Design review of the part built by this model. Coordinates are the model's own, in mm. A direction names the side the tool comes from. Give positions to 0.01 mm unless a question says otherwise; leave off trailing zeros. Write each loop counter-clockwise with the first axis right and the second up, starting at its lowest first coordinate (ties: lowest second). Pieces come first, ordered by that corner, then holes. Notation, with made-up numbers: (13.25, 69.5) -> (31.25, 69.5) arc R17 cw to (31.25, 90.5) -> close; hole circle Ø8 at (65.5, 25). An arc over 180 degrees is marked (long way). Answer as a JSON object with one key per item and string values.
```python
from build123d import *


with BuildPart() as part:
    # Sweep2: sweep along a path in BasketRing
    with BuildLine(Plane.XY) as sweep2_path:
        Line((44, 0), (273.5, 0))
        ThreePointArc((273.5, 0), (304.612698372, 12.887301628), (317.5, 44))
        Line((317.5, 44), (317.5, 203.5))
        ThreePointArc((317.5, 203.5), (304.612698372, 234.612698372), (273.5, 247.5))
        Line((273.5, 247.5), (44, 247.5))
        ThreePointArc((44, 247.5), (12.887301628, 234.612698372), (0, 203.5))
        Line((0, 203.5), (0, 44))
        ThreePointArc((0, 44), (12.887301628, 12.887301628), (44, 0))
    # ShapeOf Edge → Sweep2 (sweep)
    with BuildSketch(Plane(origin=(44, 0, 0), x_dir=(0, 0, -1), z_dir=(1, 0, 0))):
        Polygon((0, 0), (2.4, 0), (2.4, -2.4), (70.4, -2.4), (70.4, 0), (5.854935695, 0), (2.748344754, 3), (0, 3), align=None)
    sweep(path=sweep2_path.line)


solid = part.part
```
(1) The part is to be moulded in two halves that separate along X. For faces 1 (the conical face through (15.227, 232.913, -2.899)), 2 (the cylindrical face through (304.27, 12.55, -37.68)), 3 (the flat face through (-2.4, 123, -36)), 4 (the cylindrical face through (304.95, 234.27, -1.22)), say which applies: +X half, -X half, draft (parallel to the pull), parting line (faces both ways), or undercut.
Here are the results:
{"face 1": "undercut", "face 2": "undercut", "face 3": "-X half", "face 4": "+X half"}
(2) We need section A-A, the plane y = 58.5. State the section outline as (x, z) points.
Here are the results:
{"outline": "(-2.4, -70.4) -> (0, -70.4) -> (0, -5.85) -> (3, -2.75) -> (3, 0) -> (0, 0) -> (0, -2.4) -> (-2.4, -2.4) -> close; (314.5, -2.75) -> (317.5, -5.85) -> (317.5, -70.4) -> (319.9, -70.4) -> (319.9, -2.4) -> (317.5, -2.4) -> (317.5, 0) -> (314.5, 0) -> close"}
(3) For faces 5 (the cylindrical face through (12.55, 13.23, -1.22)), 6 (the cylindrical face through (14.69, 15.33, -1.35)), 7 (the flat face through (160, 0, -39)), list the 3-axis set-ups (+Z, -Z, +X, -X, +Y, -Y) from which the entire face can be reached by the end or side of a thin tool; tool diameter is ignored.
Here are the results:
{"face 5": "+Z, -X, -Y", "face 6": "+Z, -Z", "face 7": "-Z"}
(4) Clearance check with flat-ended pins moving along their axes: pin 1 (0.7 mm diameter, centred on x = 125, z = -0.5, fed in from +Y); pin 2 (1.5 mm diameter, centred on y = 207.5, z = -61, fed in from -X); pin 3 (3 mm diameter, centred on y = 207, z = -29, fed in from -X). State where each tip first meets the part, or that it passes through.
Here are the results:
{"pin 1": "stops at y = 247.5", "pin 2": "stops at x = -2.29", "pin 3": "stops at x = -2.36"}
(5) We need section C-C, the plane z = -11. State the section outline as (x, y) points.
Here are the results:
{"outline": "(-2.4, 44) arc R46.4 ccw to (44, -2.4) -> (273.5, -2.4) arc R46.4 ccw to (319.9, 44) -> (319.9, 203.5) arc R46.4 ccw to (273.5, 249.9) -> (44, 249.9) arc R46.4 ccw to (-2.4, 203.5) -> close; hole (0, 44) arc R44 ccw to (44, 0) -> (273.5, 0) arc R44 ccw to (317.5, 44) -> (317.5, 203.5) arc R44 ccw to (273.5, 247.5) -> (44, 247.5) arc R44 ccw to (0, 203.5) -> close"}
(6) We need section B-B, the plane x = 169. State the section outline as (y, z) points.
Here are the results:
{"outline": "(-2.4, -70.4) -> (0, -70.4) -> (0, -5.85) -> (3, -2.75) -> (3, 0) -> (0, 0) -> (0, -2.4) -> (-2.4, -2.4) -> close; (244.5, -2.75) -> (247.5, -5.85) -> (247.5, -70.4) -> (249.9, -70.4) -> (249.9, -2.4) -> (247.5, -2.4) -> (247.5, 0) -> (244.5, 0) -> close"}
(7) For line 1 along X through (y, z) = (146, -9); line 2 along Y through (x, z) = (227.5, -22.5); line 3 along Y through (x, z) = (167.5, -4), list the stretches that pass through material, from the lowest coordinate up.
Here are the results:
{"line 1": "x = -2.4 to 0, 317.5 to 319.9", "line 2": "y = -2.4 to 0, 247.5 to 249.9", "line 3": "y = -2.4 to 1.79, 245.71 to 249.9"}
